Design review of the part built by this model. Coordinates are the model's own, in mm. Face numbers are marked on the shaded views. A direction names the side the tool comes from. Give positions to 0.01 mm unless a question says otherwise; leave off trailing zeros. Loops run counter-clockwise (first coordinate to the right, second up) from the corner with the lowest first, then second, coordinate; pieces in that order, holes last. Notation, with made-up numbers: (-20, 46) -> (6, 46) arc R27 ccw to (6, 63) -> close; hole circle Ø5 at (-12, 49.5). An arc over 180 degrees is marked (long way). Answer as CSV lines item,"result".
from build123d import *

# Parameters (mm, degrees)
SKETCH001_W  = 53
SKETCH001_H  = 40
PAD001_DEPTH = 25
SKETCH002_R  = 5
PAD002_DEPTH = 10
SKETCH003_R  = 2.5
SKETCH003_W  = 11
SKETCH003_H  = 7
PAD003_DEPTH = 10


with BuildPart() as part:
    # Sketch001 → Pad001 (new body)
    with BuildSketch(Plane.XY):
        Rectangle(SKETCH001_W, SKETCH001_H)
    extrude(amount=PAD001_DEPTH)

    # Sketch002 (on Face2 of Pad001) → Pad002 (join)
    with BuildSketch(Plane.YZ.offset(26.5)):
        with Locations((0, 13)):
            Circle(SKETCH002_R)
    extrude(amount=PAD002_DEPTH)

    # Sketch003 (on Face2 of Pad002) → Pad003 (join)
    with BuildSketch(Plane(origin=(-26.5, 0, 0), x_dir=(0, -1, 0), z_dir=(-1, 0, 0))):
        with Locations((-5.5, 10)):
            Circle(SKETCH003_R)
        with Locations((4, 9)):
            Rectangle(SKETCH003_W, SKETCH003_H)
    extrude(amount=PAD003_DEPTH)


with BuildPart() as part_1:
    # Body001 placement: moved
    add(part.part.moved(Location((0, 0, 6))))


solid = part_1.part
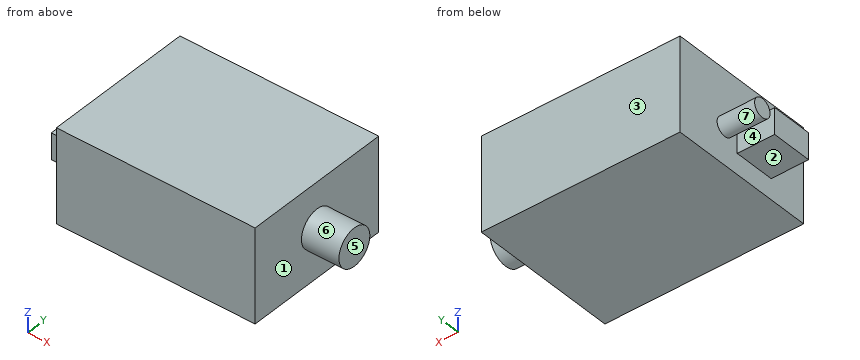
Q1. We need section B-B, the plane y = 0. State the section outline as (x, z) points.
Filled sheet:
outline,"(-36.5, 11.5) -> (-26.5, 11.5) -> (-26.5, 6) -> (26.5, 6) -> (26.5, 14) -> (36.5, 14) -> (36.5, 24) -> (26.5, 24) -> (26.5, 31) -> (-26.5, 31) -> (-26.5, 18.5) -> (-36.5, 18.5) -> close"
Q2. We need section D-D, the plane z = 10. State the section outline as (x, y) points.
Filled sheet:
outline,"(-26.5, -20) -> (26.5, -20) -> (26.5, 20) -> (-26.5, 20) -> close"
Q3. We need section C-C, the plane y = -8.5. State the section outline as (x, z) points, and give its area (4 significant figures).
Filled sheet:
outline,"(-36.5, 11.5) -> (-26.5, 11.5) -> (-26.5, 6) -> (26.5, 6) -> (26.5, 31) -> (-26.5, 31) -> (-26.5, 18.5) -> (-36.5, 18.5) -> close"
area,"1,395 mm^2"
Q4. Clearance check with flat-ended pins moving along their axes: pin 1 Ø6 at (y, z) = (7.5, 25.5) entering from -X; pin 2 Ø5.5 at (x, z) = (-29.5, 16.5) entering from -Y; pin 3 Ø11 at (x, y) = (-31.5, -3) entering from +Z; pin 4 Ø11 at (x, y) = (-32.5, -1.5) entering from -Z. State where each tip first meets the part, or that it passes through.
Filled sheet:
pin 1,"stops at x = -26.5"
pin 2,"stops at y = -9.5"
pin 3,"stops at z = 31"
pin 4,"stops at z = 11.5"
Q5. We need section A-A, the plane z = 16. State the section outline as (x, y) points.
Filled sheet:
outline,"(-36.5, -9.5) -> (-26.5, -9.5) -> (-26.5, -20) -> (26.5, -20) -> (26.5, -4) -> (36.5, -4) -> (36.5, 4) -> (26.5, 4) -> (26.5, 20) -> (-26.5, 20) -> (-26.5, 8) -> (-36.5, 8) -> (-36.5, 3) -> (-26.5, 3) -> (-26.5, 1.5) -> (-36.5, 1.5) -> close"
Q6. The part is to be moulded in two halves that separate along Y. For the marked faces 4, 5, 6 and 7, say which applies: pulls with the +Y half, pulls with the -Y half, needs draft (parallel to the pull), parting line crosses it, or undercut.
Filled sheet:
face 4,"undercut"
face 5,"needs draft"
face 6,"parting line crosses it"
face 7,"undercut"
Q7. To check wall thickness, follow probe 1 along Y at (x, z) = (-32, 15.75); probe 2 along X at (y, z) = (-12.5, 25.5); probe 3 along X at (y, z) = (-3.5, 19.5). State the ranges of each line that lie inside material, in increasing order. Write a range as from..to.
Filled sheet:
probe 1,"y = -9.5..1.5, 3.01..7.99"
probe 2,"x = -26.5..26.5"
probe 3,"x = -26.5..36.5"
Q8. For the marked faces 1, 2 and 3, list the 3-axis set-ups (+Z, -Z, +X, -X, +Y, -Y) from which the entire face can be reached by the end or side of a thin tool; tool diameter is ignored.
Filled sheet:
face 1,"+X"
face 2,"-Z, -X, +Y, -Y"
face 3,"+Z, -Z, +X, -X, +Y"
